The listing builds one solid part. Answer for the finished solid, in the listing's coordinates (mm). A direction names the side the tool comes from. Round coordinates to 2 decimals unless told otherwise and drop trailing zeros. Write each loop counter-clockwise with the first axis right and the second up, starting at its lowest first coordinate (ties: lowest second). Pieces come first, ordered by that corner, then holes.
from build123d import *

# Parameters (mm, degrees)
SKETCH2_W           = 44
SKETCH2_H           = 44
BOSS_EXTRUDE1_DEPTH = 2
SKETCH4_W           = 10.31875
SKETCH4_H           = 8
CUT_EXTRUDE1_DEPTH  = 32.176914536
SKETCH5_R           = 0.4
CUT_EXTRUDE2_DEPTH  = 3
SKETCH8_W           = 2
SKETCH8_H           = 44
BOSS_EXTRUDE2_DEPTH = 35
SKETCH11_R          = 1.143
SKETCH11_R_2        = 1.15
CUT_EXTRUDE3_DEPTH  = 10
FILLET1_R           = 10
SKETCH14_R          = 4.351447522
SKETCH14_R_2        = 4.637760651
SKETCH14_R_3        = 2.653670008
CUT_EXTRUDE5_DEPTH  = 10
LPATTERN1_COUNT     = 3
LPATTERN1_PITCH     = 13
SKETCH16_R          = 3.212197925
SKETCH16_R_2        = 3.154230468
SKETCH16_R_3        = 3.167930334
SKETCH16_R_4        = 3.203393346
CUT_EXTRUDE6_DEPTH  = 10


with BuildPart() as part:
    # Sketch2 → Boss-Extrude1 (new body)
    with BuildSketch(Plane(origin=(0, 0, 0), x_dir=(1, 0, 0), z_dir=(0, 1, 0))):
        Rectangle(SKETCH2_W, SKETCH2_H)
    extrude(amount=BOSS_EXTRUDE1_DEPTH)

    # Sketch4 → Cut-Extrude1 (cut, through all)
    with BuildSketch(Plane.XZ):
        Rectangle(SKETCH4_W, SKETCH4_H)
    extrude(amount=-CUT_EXTRUDE1_DEPTH, mode=Mode.SUBTRACT)

    # Sketch5 → Cut-Extrude2 (cut)
    with BuildSketch(Plane.XZ):
        with Locations(Location((-11.5, 0, 0), (0, 0, 270))):
            Circle(SKETCH5_R)
    cut_extrude2 = extrude(amount=-CUT_EXTRUDE2_DEPTH, mode=Mode.SUBTRACT)

    # Mirror1: Cut-Extrude2 across plane
    add(cut_extrude2.mirror(Plane(origin=(0, 0, 0), x_dir=(0, 0, 1), z_dir=(1, 0, 0))), mode=Mode.SUBTRACT)

    # Sketch8 → Boss-Extrude2 (add)
    with BuildSketch(Plane(origin=(0, 2, 0), x_dir=(1, 0, 0), z_dir=(0, 1, 0))):
        with Locations((-21, 0)):
            Rectangle(SKETCH8_W, SKETCH8_H)
    boss_extrude2 = extrude(amount=BOSS_EXTRUDE2_DEPTH)

    # Mirror2: Boss-Extrude2 across plane
    add(boss_extrude2.mirror(Plane(origin=(0, 0, 0), x_dir=(0, 0, 1), z_dir=(1, 0, 0))))

    # Sketch11 → Cut-Extrude3 (cut)
    with BuildSketch(Plane.ZY.offset(22)):
        with Locations((-9.153659498, 12.053864297)):
            Circle(SKETCH11_R)
        with Locations((12.458196086, 30.478767136)):
            Circle(SKETCH11_R_2)
        Polygon((-11.290641548, 18.478237521), (-3.43872233, 9.140820073), (14.47075048, 24.201058573), (6.618831262, 33.538476021), align=None)
    extrude(amount=-CUT_EXTRUDE3_DEPTH, mode=Mode.SUBTRACT)

    # Fillet1
    fillet1_edges = [part.edges().sort_by_distance(p)[0] for p in [
        (-21, 37, 22),
        (-21, 37, -22),
        (21, 37, -22),
        (21, 37, 22),
    ]]
    fillet(fillet1_edges, radius=FILLET1_R)

    # Sketch14 → Cut-Extrude5 (cut)
    with BuildSketch(Plane(origin=(22, 0, 0), x_dir=(0, 0, -1), z_dir=(1, 0, 0))):
        with Locations((-12.858925156, 29.108613253)):
            Circle(SKETCH14_R)
        with Locations((-12.858925156, 17.175691446)):
            Circle(SKETCH14_R_2)
        with Locations((-12.858925156, 6.998624266)):
            Circle(SKETCH14_R_3)
    cut_extrude5 = extrude(amount=-CUT_EXTRUDE5_DEPTH, mode=Mode.SUBTRACT)

    # LPattern1: Cut-Extrude5 ×3
    with Locations(*[(0, 0, -i * LPATTERN1_PITCH) for i in range(1, LPATTERN1_COUNT)]):
        add(cut_extrude5, mode=Mode.SUBTRACT)

    # Sketch16 → Cut-Extrude6 (cut)
    with BuildSketch(Plane(origin=(22, 0, 0), x_dir=(0, 0, -1), z_dir=(1, 0, 0))):
        with Locations((-6.443418132, 10.901979994)):
            Circle(SKETCH16_R)
        with Locations((7.118442889, 10.901979994)):
            Circle(SKETCH16_R_2)
        with Locations((7.118442889, 23.236523275)):
            Circle(SKETCH16_R_3)
        with Locations((-6.443418132, 23.236523275)):
            Circle(SKETCH16_R_4)
    extrude(amount=-CUT_EXTRUDE6_DEPTH, mode=Mode.SUBTRACT)


solid = part.part
1. Section A-A on x = 2 is taken. Determine the outline of the cut face in (y, z), plus the area to 3 significant figures.
Geometry says:
outline: (0, -22) - (2, -22) - (2, -4) - (0, -4) - close; (0, 4) - (2, 4) - (2, 22) - (0, 22) - close
area: 72.0 mm2
2. Section B-B on y = 3 is taken. Determine the outline of the cut face in (x, z), plus the area to 3 significant figures.
Geometry says:
outline: (-22, -22) - (-20, -22) - (-20, 22) - (-22, 22) - close; (20, -22) - (22, -22) - (22, 22) - (20, 22) - close
area: 176 mm2
3. Given pin 1 (5 mm diameter, centred on y = 7, z = 12.86, fed in from +X); pin 2 (1.5 mm diameter, centred on x = 16, z = -3.5, fed in from +Y), each flat-ended and moving along its own axis, determine where each tip first touches the part or whether it passes through.
Geometry says:
pin 1: stops at x = -20
pin 2: stops at y = 2
4. Straight lines are drawn through the part: line 1 along X through (y, z) = (1, 0); line 2 along X through (y, z) = (4, 19); line 3 along X through (y, z) = (30.5, -4). For each, find the intervals that lie inside material, in ascending order.
Geometry says:
line 1: x = -22 to -11.9, -11.1 to -5.16, 5.16 to 11.1, 11.9 to 22
line 2: x = -22 to -20, 20 to 22
line 3: x = -22 to -20
5. Section C-C on z = -1 is taken. Determine the outline of the cut face in (x, y), plus the area to 3 significant figures.
Geometry says:
outline: (-22, 0) - (-5.16, 0) - (-5.16, 2) - (-20, 2) - (-20, 11.19) - (-22, 11.19) - close; (-22, 27.13) - (-20, 27.13) - (-20, 37) - (-22, 37) - close; (5.16, 0) - (22, 0) - (22, 4.49) - (20, 4.49) - (20, 2) - (5.16, 2) - close; (20, 9.51) - (22, 9.51) - (22, 12.62) - (20, 12.62) - close; (20, 21.73) - (22, 21.73) - (22, 24.84) - (20, 24.84) - close; (20, 33.37) - (22, 33.37) - (22, 37) - (20, 37) - close
area: 130 mm2
6. Section D-D on x = -10 is taken. Determine the outline of the cut face in (y, z), plus the area to 3 significant figures.
Geometry says:
outline: (0, -22) - (2, -22) - (2, 22) - (0, 22) - close
area: 88.0 mm2
7. For a pull along Z with two mould halves and no side action, classify faces 6 (the face through (21.014, 21.774, 0.463)), 7 (the face through (20.99, 34.15, -18.99)), 8 (the face through (-21, 37, 0)) as released by +Z, released by -Z, zero draft, split by the parting line, or undercut.
Geometry says:
face 6: undercut
face 7: released by -Z
face 8: zero draft
8. A tool of negligible diameter and unlimited length cuts with its end or side. For faces 1 (the face through (21.014, 20.426, -8.58)), 2 (the face through (-21.014, 29.356, 12.209)), 3 (the face through (-21.014, 28.804, 10.6)), 4 (the face through (2, 1, -22)), 5 (the face through (20, 19, 5)), from which of +Z, -Z, +X, -X, +Y, -Y can it reach the whole face along a straight path? Write none if from no direction.
Geometry says:
face 1: +X
face 2: +X, -X
face 3: -X
face 4: -Z, +X, -X, +Y, -Y
face 5: +Z, -Z, +Y
